CAD build for the part. Positions are in the model's coordinates, mm. A direction names the side the tool comes from. Give positions to 0.01 mm unless a question says otherwise; leave off trailing zeros. Loops run counter-clockwise (first coordinate to the right, second up) from the corner with the lowest first, then second, coordinate; pieces in that order, holes last. Notation, with made-up numbers: (88, 53.5) - (133, 53.5) arc R27 ccw to (133, 78.5) - close; hole circle Ø5 at (5, -19). An arc over 180 degrees is marked (long way). Return JSON: item names as keys, results as strings.
Autodesk Inventor part; units mm, degrees
ref_plane "Work Plane1" through (29, 0, 0) normal (0, -1, 0) x (1, 0, 0)
ref_plane "YZ Plane" through (0, 0, 0) normal (1, 0, 0) x (0, 1, 0)
ref_plane "XZ Plane" through (0, 0, 0) normal (0, 1, 0) x (-1, 0, 0)
sketch "Sketch1" plane through (0, 0, 0) normal (0, 0, 1) x (1, 0, 0)
  line L0 (-1.1667, 0) -> (120, 0)
  line L1 (120, 0) -> (120, 2.5)
  line L2 (120, 2.5) -> (98, 2.5)
  line L3 (98, 2.5) -> (97.5091, 2.5)
  line L4 (97.5091, 2.5) -> (0, 2.5)
  line L5 (0, 2.5) -> (0, 4.25)
  line L6 (0, 4.25) -> (-5, 4.25)
  line L7 (-5, 4.25) -> (-5, 2.3094)
  line L8 (-5, 2.3094) -> (-2.5, 2.3094)
  line L9 (-2.5, 2.3094) -> (-1.1667, 0)
  line L10 (-22, 0) -> (97, 0)
  line L11 (0, -0.85) -> (0, 5.1)
  line L12 (98, 2.5) -> (0, 2.5) construction
  dimension "d1" = 22
  dimension "d2" = 0.4909
  dimension "d3" = 5
  dimension "d4" = 2.5
  dimension "d5" = 60
  dimension "d6" = 5
  dimension "d7" = 5
  dimension "d8" = 4.6188
  dimension "d9" = 8.5
  dimension "d26" = 120
revolve "Body" add sketch "Sketch1" angle 360 about axis through (-1.1667, 0, 0) along (1, 0, 0)
sketch "Sketch2" plane through (-5, 0, 0) normal (-1, 0, 0) x (0, 0, 1)
  circle A0 centre (0, 0) radius 2.3094
  line L0 (0, -5.95) -> (0, 5.95)
  line L1 (-5.95, 0) -> (5.95, 0)
  line L2 (2.3094, 0) -> (1.1547, -2)
  line L3 (1.1547, -2) -> (-1.1547, -2)
  line L4 (-1.1547, -2) -> (-2.3094, 0)
  line L5 (-2.3094, 0) -> (-1.1547, 2)
  line L6 (-1.1547, 2) -> (1.1547, 2)
  line L7 (1.1547, 2) -> (2.3094, 0)
extrude "Slot" add sketch "Sketch2" against normal up to next contours L7 A0 | A0 L2 | L6 L0 A0 | A0 L0 L3 | L0 L6 A0 | A0 L3 L0 | L4 A0 | A0 L5
fillet "Fillet1" radius 0.5 1 edges at (-5, -4.25, 0)
thread "Thread"
chamfer "Chamfer1" distance 0.4908 distance2 0.4908 1 edges at (120, -2.5, 0) measured on face at (120, -0.6238, 0.5526)
ref_plane "Work Plane1" through (29, 0, 0) normal (0, -1, 0) x (1, 0, 0)
fillet "Fillet2" radius 0.2 1 edges at (0, -2.5, 0)
equation "\"d30\" = R"
equation "\"d17\" = RR"
equation "\"d13\" = GEL"
equation "\"d15\" = -0.5 * SPD + 0.5 * GD"
equation "\"d16\" = GUL"
equation "\"d1\" = GEL"
equation "\"d3\" = KOH"
equation "\"d4\" = INTI"
equation "\"d6\" = GD"
equation "\"d7\" = BDM"
equation "\"d8\" = 1.1547 * SW"
equation "\"d9\" = KOD"
equation "\"d26\" = NLG"
equation "\"GD\" = NND"
equation "\"NLG\" = 120"
equation "\"GEL\" = 22"
equation "\"KOD\" = 8.5"
equation "\"KOH\" = 5"
equation "\"INTI\" = 2.5"
equation "\"GAL\" = 0.61345 * PTC"
equation "\"GUL\" = 0.61345 * PTC"
equation "\"BDM\" = NND"
equation "\"SW\" = 4"
equation "\"RR\" = 0.5"
equation "\"SPD\" = NND - 1.2269 * PTC"
equation "\"R\" = 0.2"
equation "\"TOA\" = 30deg"
equation "\"GD1\" = THREADDIA - 1.2269 * PTC"
equation "\"THREADDIA\" = 5"
equation "\"FAWI\" = 45deg"
equation "\"ANG\" = 120deg"
equation "\"PTC\" = 0.8"
equation "\"NND\" = 5"
equation "\"E0\" = 1.155 * SW"
properties material "Steel, Mild"
1. Cut at A-A, the plane x = 72. Write the cut outline in (y, z).
Values follow:
{"outline": "circle Ø5 at (0, 0)"}
2. Which spindle directions (+Z, -Z, +X, -X, +Y, -Y) get a long thin tool onto all of the face, cutting with end or side? Do faces 1 (the face through (0, 0, -3)), 2 (the face through (-3.679, -1.014, -1.724)), 3 (the face through (120, 0, 0)). Say none if no direction does.
Values follow:
{"face 1": "+X", "face 2": "-X", "face 3": "+Z, -Z, +X, +Y, -Y"}
3. Drill centre lines: probe 1 along X at (y, z) = (-1.75, -3.25); probe 2 along Y at (x, z) = (22.5, -1). Where is each one in solid material? Low to high.
Values follow:
{"probe 1": "x = -5 to 0", "probe 2": "y = -2.29 to 2.29"}
4. Drop flat-ended pins along their axis: P1, Ø1, axis at x = 57.5, y = 2, coming from the -Z side; P2, Ø3, axis at x = 72.5, z = -2.5, coming from the -Y side; P3, Ø1.5, axis at y = -2, z = -2, coming from the +X side; P4, Ø5, axis at y = -2.5, z = 3.5, coming from the +X side. Give the stop position or say it passes through.
Values follow:
{"P1": "stops at z = -2", "P2": "stops at y = -2.29", "P3": "stops at x = 119.93", "P4": "stops at x = 120"}
